from build123d import *

# Parameters (mm, degrees)
SKETCH1_W           = 101.6
SKETCH1_H           = 50
BOSS_EXTRUDE1_DEPTH = 6.35
SKETCH3_W           = 6.35
SKETCH3_H           = 25
CUT_EXTRUDE2_DEPTH  = 7.35
SKETCH4_W           = 6.35
SKETCH4_H           = 25
SKETCH4_W_2         = 50
SKETCH4_H_2         = 6.35
CUT_EXTRUDE3_DEPTH  = 7.35


with BuildPart() as part:
    # Sketch1 → Boss-Extrude1 (new body)
    with BuildSketch(Plane.XY):
        with Locations((50.8, 25)):
            Rectangle(SKETCH1_W, SKETCH1_H)
    extrude(amount=BOSS_EXTRUDE1_DEPTH)

    # Sketch3 → Cut-Extrude2 (cut, through all)
    with BuildSketch(Plane.XY.offset(6.35)):
        with Locations((3.175, 25)):
            Rectangle(SKETCH3_W, SKETCH3_H)
    extrude(amount=-CUT_EXTRUDE2_DEPTH, mode=Mode.SUBTRACT)

    # Sketch4 → Cut-Extrude3 (cut, through all)
    with BuildSketch(Plane.XY.offset(6.35)):
        with Locations((98.425, 25)):
            Rectangle(SKETCH4_W, SKETCH4_H)
        with Locations((51.6, 46.825)):
            Rectangle(SKETCH4_W_2, SKETCH4_H_2)
        with Locations((51.6, 3.175)):
            Rectangle(SKETCH4_W_2, SKETCH4_H_2)
    extrude(amount=-CUT_EXTRUDE3_DEPTH, mode=Mode.SUBTRACT)


solid = part.part
Verification items for the finished model (mm, model axes). A direction names the side the tool comes from. Give positions to 0.01 mm unless a question says otherwise; leave off trailing zeros. Write each loop counter-clockwise with the first axis right and the second up, starting at its lowest first coordinate (ties: lowest second). Pieces come first, ordered by that corner, then holes.
(1) Access from +Z, -Z, +X, -X, +Y, -Y to the whole of each face (thin tool, end or side, straight path). Record for faces 1 (the face through (3, 37.5, 3)), 2 (the face through (26.6, 47, 3)), 3 (the face through (26.6, 3, 3)).
(2) Cross-section at B-B (x = 70.5). Enter the section's corners in (y, z), plus the area to 3 significant figures.
(3) Cross-section at A-A (z = 4.25). Enter the section's corners in (x, y).
(4) Material ranges on line 1 (Y direction, x = 97, z = 2); line 2 (X direction, y = 4, z = 2); line 3 (X direction, y = 28.5, z = 3.25), recorded low to high.
(5) Cross-section at C-C (y = 34). Enter the section's corners in (x, z).
(6) Mould release check, pull along Y, two halves, no side actions. Record for faces 4 (the face through (51, 43.65, 3)), 5 (the face through (76.6, 3, 3)), 6 (the face through (3, 12.5, 3)), 7 (the face through (13, 0, 3)): +Y half, -Y half, draft (parallel to the pull), parting line (faces both ways), or undercut.
(7) Gauge pin test, flat ends, axial feed: pin 1 (4 mm diameter, centred on x = 53, y = 20, fed in from -Z); pin 2 (1.9 mm diameter, centred on x = 53.5, z = 3, fed in from -Y); pin 3 (3 mm diameter, centred on y = 26, z = 2, fed in from +X). Record the tip position at first contact, or that the pin passes through.
Worked out:
1. face 1: +Z, -Z, -X
1. face 2: +Z, -Z, +Y
1. face 3: +Z, -Z, -Y
2. outline: (6.35, 0) - (43.65, 0) - (43.65, 6.35) - (6.35, 6.35) - close
2. area: 237 mm2
3. outline: (0, 0) - (26.6, 0) - (26.6, 6.35) - (76.6, 6.35) - (76.6, 0) - (101.6, 0) - (101.6, 12.5) - (95.25, 12.5) - (95.25, 37.5) - (101.6, 37.5) - (101.6, 50) - (76.6, 50) - (76.6, 43.65) - (26.6, 43.65) - (26.6, 50) - (0, 50) - (0, 37.5) - (6.35, 37.5) - (6.35, 12.5) - (0, 12.5) - close
4. line 1: y = 0 to 12.5, 37.5 to 50
4. line 2: x = 0 to 26.6, 76.6 to 101.6
4. line 3: x = 6.35 to 95.25
5. outline: (6.35, 0) - (95.25, 0) - (95.25, 6.35) - (6.35, 6.35) - close
6. face 4: +Y half
6. face 5: draft
6. face 6: undercut
6. face 7: -Y half
7. pin 1: stops at z = 0
7. pin 2: stops at y = 6.35
7. pin 3: stops at x = 95.25
